For this review, take the finished solid that the model builds, in its own axes (mm). Face numbers are marked on the shaded views. A direction names the side the tool comes from. Round coordinates to 2 decimals unless told otherwise and drop trailing zeros. Order: outer loops, then holes, each group sorted by start corner. A loop starts at its lowest first (then second) coordinate and runs counter-clockwise, first axis right, second up. Notation, with made-up numbers: M 51,-8 L 57,-8 A11 cw 57,8 Z; hole C -33,64 d9. An arc over 180 degrees is marked long. Answer as a JSON object with one key per item and string values.
from build123d import *

# Parameters (mm, degrees)
SKETCH1_W           = 84
SKETCH1_H           = 48
BOSS_EXTRUDE1_DEPTH = 0.8
SKETCH2_R           = 1.6
CUT_EXTRUDE1_DEPTH  = 49.4
SKETCH3_W           = 6.862119169
SKETCH3_H           = 27.332124702
SKETCH3_W_2         = 10.110629261
SKETCH3_H_2         = 3.312844108
SKETCH3_W_3         = 9.995650326
SKETCH3_H_3         = 6.943369618
SKETCH3_W_4         = 11.50293093
SKETCH3_H_4         = 17.135400557
SKETCH3_H_5         = 15.193388494
SKETCH3_W_5         = 8.420598576
SKETCH3_H_6         = 36.987675992
BOSS_EXTRUDE2_DEPTH = 10


with BuildPart() as part:
    # Sketch1 → Boss-Extrude1 (new, symmetric)
    with BuildSketch(Plane.XY):
        Rectangle(SKETCH1_W, SKETCH1_H)
    extrude(amount=BOSS_EXTRUDE1_DEPTH, both=True)

    # Sketch2 → Cut-Extrude1 (cut, through all)
    with BuildSketch(Plane.XY.offset(0.8)):
        with Locations((-39, -21)):
            Circle(SKETCH2_R)
        with Locations((-39, 21)):
            Circle(SKETCH2_R)
        Circle(SKETCH2_R)
        with Locations((39, -21)):
            Circle(SKETCH2_R)
        with Locations((39, 21)):
            Circle(SKETCH2_R)
    extrude(amount=-CUT_EXTRUDE1_DEPTH, mode=Mode.SUBTRACT)

    # Sketch3 → Boss-Extrude2 (add)
    with BuildSketch(Plane.XY.offset(0.8)):
        with Locations((-31.966191102, -3.002126176)):
            Rectangle(SKETCH3_W, SKETCH3_H)
        with Locations((-13.456350493, 17.232506389)):
            Rectangle(SKETCH3_W_2, SKETCH3_H_2)
        with Locations((-0.93444373, 18.273143727)):
            Rectangle(SKETCH3_W_3, SKETCH3_H_3)
        with Locations((-20.403749308, -12.069028564)):
            Rectangle(SKETCH3_W_4, SKETCH3_H_4)
        with Locations((-20.403749308, 5.009253991)):
            Rectangle(SKETCH3_W_4, SKETCH3_H_5)
        with Locations((31.938626633, 0.080507911)):
            Rectangle(SKETCH3_W_5, SKETCH3_H_6)
    extrude(amount=BOSS_EXTRUDE2_DEPTH)


solid = part.part
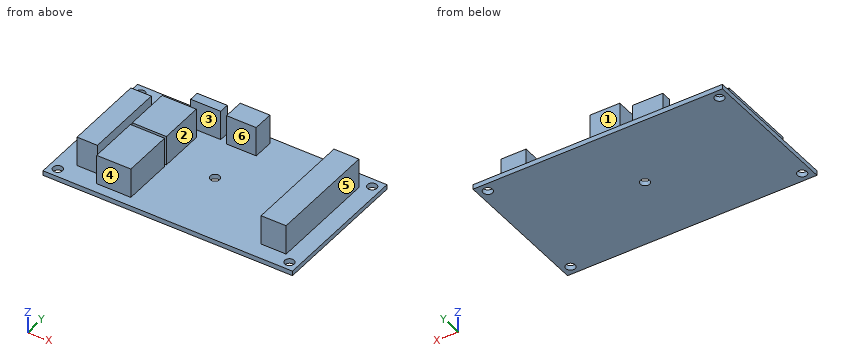
1) Mouldability with a two-part tool opening along Y and no side actions: class the marked faces 1, 2 and 3 as +Y half, -Y half, draft (parallel to the pull), parting line (faces both ways), or undercut.
Geometry check:
{"face 1": "+Y half", "face 2": "draft", "face 3": "undercut"}
2) Insertion check: P1, Ø5, axis at y = 3.5, z = 4, coming from the +X side; P2, Ø5, axis at y = 0.5, z = 5.5, coming from the -X side; P3, Ø3.5, axis at y = 17, z = 8, coming from the -X side. Each pin has a flat end and moves straight along its axis. Give the tip position at first contact, or say it passes through.
Geometry check:
{"P1": "stops at x = 36.15", "P2": "stops at x = -35.4", "P3": "stops at x = -18.51"}
3) Machinability: for the marked faces 4, 5 and 6, which of the approach directions +Z, -Z, +X, -X, +Y, -Y give a long, thin tool a straight path to every point of the face, cutting with its end or side? Answer none if there is none.
Geometry check:
{"face 4": "+Z, +X, -X, -Y", "face 5": "+Z, +X, +Y, -Y", "face 6": "+Z, -X, -Y"}
4) For L1, parallel to Y at x = -17.5, z = 1.75; L2, parallel to X at y = 10.5, z = 6.75; L3, parallel to Y at x = 39, z = 0.5, list the stretches that pass through material, from the lowest coordinate up.
Geometry check:
{"L1": "y = -20.64 to -3.5, -2.59 to 12.61, 15.58 to 18.89", "L2": "x = -35.4 to -28.54, -26.16 to -14.65, 27.73 to 36.15", "L3": "y = -24 to -22.6, -19.4 to 19.4, 22.6 to 24"}
5) Add section A-A on x = 0. State the section outline as (y, z) points, and give its area (3 significant figures).
Geometry check:
{"outline": "M -24,-0.8 L -1.6,-0.8 L -1.6,0.8 L -24,0.8 Z; M 1.6,-0.8 L 24,-0.8 L 24,0.8 L 21.74,0.8 L 21.74,10.8 L 14.8,10.8 L 14.8,0.8 L 1.6,0.8 Z", "area": "141 mm²"}
6) Add section C-C on x = 39. State the section outline as (y, z) points.
Geometry check:
{"outline": "M -24,-0.8 L -22.6,-0.8 L -22.6,0.8 L -24,0.8 Z; M -19.4,-0.8 L 19.4,-0.8 L 19.4,0.8 L -19.4,0.8 Z; M 22.6,-0.8 L 24,-0.8 L 24,0.8 L 22.6,0.8 Z"}
7) Add section D-D on y = -6. State the section outline as (x, z) points.
Geometry check:
{"outline": "M -42,-0.8 L 42,-0.8 L 42,0.8 L 36.15,0.8 L 36.15,10.8 L 27.73,10.8 L 27.73,0.8 L -14.65,0.8 L -14.65,10.8 L -26.16,10.8 L -26.16,0.8 L -28.54,0.8 L -28.54,10.8 L -35.4,10.8 L -35.4,0.8 L -42,0.8 Z"}
8) Add section B-B on z = 9.5. State the section outline as (x, y) points.
Geometry check:
{"outline": "M -35.4,-16.67 L -28.54,-16.67 L -28.54,10.66 L -35.4,10.66 Z; M -26.16,-20.64 L -14.65,-20.64 L -14.65,-3.5 L -26.16,-3.5 Z; M -26.16,-2.59 L -14.65,-2.59 L -14.65,12.61 L -26.16,12.61 Z; M -18.51,15.58 L -8.4,15.58 L -8.4,18.89 L -18.51,18.89 Z; M -5.93,14.8 L 4.06,14.8 L 4.06,21.74 L -5.93,21.74 Z; M 27.73,-18.41 L 36.15,-18.41 L 36.15,18.57 L 27.73,18.57 Z"}
